Check sheet for the modelled part. Datum: model origin and axes. Units: mm. A direction names the side the tool comes from. Round coordinates to 2 decimals unless told otherwise and drop trailing zeros. Order: outer loops, then holes, each group sorted by start corner. A loop starts at its lowest first (then second) coordinate and runs counter-clockwise, first axis right, second up. Notation, with made-up numbers: (-4, 13.25) -> (46, 13.25) arc R19 ccw to (46, 17.25) -> close; hole circle Ø10 at (43, -32). An arc over 180 degrees is marked (long way). Answer in a Markdown table with one row per item. Add a question column.
1. Sectioned sample at A-A, the plane y = 40. Record the boundary of the cut face in (x, z).
2. Material ranges on L1, parallel to X at y = 39, z = 0; L2, parallel to Y at x = 2.5, z = 2.75, recorded low to high. Write a range as from..to.
3. Access from +Z, -Z, +X, -X, +Y, -Y to the whole of each face (thin tool, end or side, straight path). Record for faces 5 (the cylindrical face through (2.287, 0.256, -3.434)), 6 (the cylindrical face through (-0.867, 77.644, 3.905)), 7 (the cylindrical face through (-3.746, 78.397, -0.165)), 8 (the cylindrical face through (2.42, 3.03, 2.76)).
4. Draft check along Z on faces 1 (the cylindrical face through (-0.867, 81.264, 3.905)), 2 (the flat face through (2, 3, -2.7)), 3 (the cylindrical face through (1.99, 2.56, 2.76)), 4 (the cylindrical face through (-0.163, 4.268, 3.812)). Enter one of: +Z half, -Z half, draft (parallel to the pull), parting line (faces both ways), or undercut.
5. Depth check by flat-ended pin: P1, Ø4, axis at x = -3.5, z = 2.5, coming from the +Y side; P2, Ø0.8, axis at x = 2, y = 3, coming from the -Z side; P3, Ø5, axis at y = 37.5, z = -0.5, coming from the -X side. Enter the tip coordinate at first touch or a pass-through.
```python
from build123d import *

# Parameters (mm, degrees)
ESQUISSE3_W                  = 7.5
ESQUISSE3_H                  = 5.8
ENL_V_MAT_EXTRU_1_DEPTH      = 8
CONG_1_R                     = 0.5
ENL_V_MAT_EXTRU_2_DEPTH      = 89.206964432
ENL_V_MAT_EXTRU_2_DEPTH_BACK = 89.206964432
ESQUISSE4_R                  = 0.75
ESQUISSE5_W                  = 0.75
ESQUISSE5_H                  = 3.75
ESQUISSE5_W_2                = 2.511980861
ESQUISSE5_H_2                = 0.75
BOSS_EXTRU_1_DEPTH           = 0.2
CONG_2_R                     = 0.2
CONG_2_OF_SYM_TRIE1_R        = 0.2
ENL_V_MAT_EXTRU_3_DEPTH      = 89.410568231


with BuildPart() as part:
    # Esquisse2 → Révolution1 (revolve)
    with BuildSketch(Plane.XY):
        with BuildLine():
            Line((4.014003451, 30.213287326), (4.735996549, 20.586712674))
            ThreePointArc((4.735996549, 20.586712674), (4.746497911, 20.399868856), (4.75, 20.212762933))
            Line((4.75, 20.212762933), (4.75, 0))
            Line((4.75, 0), (1, 0))
            Line((1, 0), (1, 83.950802))
            Line((1, 83.950802), (0, 83.950802))
            Line((0, 83.950802), (0, 87.950802))
            ThreePointArc((0, 87.950802), (2.828427125, 86.779229125), (4, 83.950802))
            Line((4, 83.950802), (4, 78.650802))
            Line((4, 78.650802), (3.75, 78.650802))
            Line((3.75, 78.650802), (3.75, 78.150802))
            Line((3.75, 78.150802), (4, 78.150802))
            Line((4, 78.150802), (4, 77.150802))
            Line((4, 77.150802), (3.75, 77.150802))
            Line((3.75, 77.150802), (3.75, 76.650802))
            Line((3.75, 76.650802), (4, 76.650802))
            Line((4, 76.650802), (4, 30.587237067))
            ThreePointArc((4, 30.587237067), (4.003502089, 30.400131144), (4.014003451, 30.213287326))
        make_face()
    revolve(axis=Axis((0, 0, 0), (0, 1, 0)))

    # Esquisse3 → Enlèv. mat.-Extru.1 (cut)
    with BuildSketch(Plane.XZ):
        with Locations((1, 0)):
            Rectangle(ESQUISSE3_W, ESQUISSE3_H)
    extrude(amount=-ENL_V_MAT_EXTRU_1_DEPTH, mode=Mode.SUBTRACT)

    # Congé1
    cong_1_edges = [part.edges().sort_by_distance(p)[0] for p in [
        (-4.75, 0, 0),
    ]]
    fillet(cong_1_edges, radius=CONG_1_R)

    # Esquisse4 → Enlèv. mat.-Extru.2 (cut, two sides: drawn at the far end of the back side and taken through both)
    with BuildSketch(Plane.XY.offset(-ENL_V_MAT_EXTRU_2_DEPTH_BACK)):
        with Locations((0, 5)):
            Circle(ESQUISSE4_R)
        with BuildLine():
            Line((1.161980861, 0), (3.761980861, 0))
            Line((3.761980861, 0), (3.761980861, 2.6))
            ThreePointArc((3.761980861, 2.6), (3.000458492, 0.761522369), (1.161980861, 0))
        make_face()
        Polygon((3.761980861, 8), (4.75, 10), (4.75, 8), align=None)
    extrude(amount=ENL_V_MAT_EXTRU_2_DEPTH + ENL_V_MAT_EXTRU_2_DEPTH_BACK, mode=Mode.SUBTRACT)

    # Esquisse5 → Boss.-Extru.1 (add)
    with BuildSketch(Plane.XY.offset(-2.9)):
        with Locations((0, 1.875)):
            Rectangle(ESQUISSE5_W, ESQUISSE5_H)
        Polygon((0.618718434, 3.850951481), (1.149048519, 4.381281566), (4.027145904, 1.503184182), (3.496815818, 0.972854096), align=None)
        with Locations((2.50599043, 5)):
            Rectangle(ESQUISSE5_W_2, ESQUISSE5_H_2)
    boss_extru_1 = extrude(amount=BOSS_EXTRU_1_DEPTH)

    # Congé2
    cong_2_edges = [part.edges().sort_by_distance(p)[0] for p in [
        (2.505990431, 5.375, -2.7),
        (2.505990431, 4.625, -2.7),
        (2.588097212, 2.942232874, -2.7),
        (2.057767126, 2.411902788, -2.7),
        (-0.375, 1.875, -2.7),
        (0.375, 1.875, -2.7),
    ]]
    fillet(cong_2_edges, radius=CONG_2_R - 0.0001)  # a hair under: the kernel refuses the full size

    # Symétrie1: Boss.-Extru.1 across plane
    add(boss_extru_1.mirror(Plane.XY))

    # Congé2 of Symétrie1
    cong_2_of_sym_trie1_edges = [part.edges().sort_by_distance(p)[0] for p in [
        (2.505990431, 5.375, 2.7),
        (2.505990431, 4.625, 2.7),
        (2.588097212, 2.942232874, 2.7),
        (2.057767126, 2.411902788, 2.7),
        (-0.375, 1.875, 2.7),
        (0.375, 1.875, 2.7),
    ]]
    fillet(cong_2_of_sym_trie1_edges, radius=CONG_2_OF_SYM_TRIE1_R - 0.0001)  # a hair under: the kernel refuses the full size

    # Esquisse6 → Enlèv. mat.-Extru.3 (cut, through all)
    with BuildSketch(Plane.XY.offset(2.9)):
        with BuildLine():
            Line((4.027145904, 1.503184182), (3.658059706, 1.87227038))
            ThreePointArc((3.658059706, 1.87227038), (3.516870908, 1.49795968), (3.319930166, 1.149739748))
            Line((3.319930166, 1.149739748), (3.496815818, 0.972854096))
            Line((3.496815818, 0.972854096), (4.027145904, 1.503184182))
        make_face()
    extrude(amount=-ENL_V_MAT_EXTRU_3_DEPTH, mode=Mode.SUBTRACT)


solid = part.part
```
Answer key:
| question | item | result |
|---|---|---|
| 1 | outline | circle Ø8 at (0, 0); hole circle Ø2 at (0, 0) |
| 2 | L1 | x = -4..-1, 1..4 |
| 2 | L2 | y = 2.07..2.93, 4.69..5.31, 8..85.43 |
| 3 | face 5 | +Z, -Z, +X, -Y |
| 3 | face 6 | +Y |
| 3 | face 7 | none |
| 3 | face 8 | +X |
| 4 | face 1 | parting line |
| 4 | face 2 | undercut |
| 4 | face 3 | undercut |
| 4 | face 4 | draft |
| 5 | P1 | stops at y = 87.22 |
| 5 | P2 | stops at z = -4.47 |
| 5 | P3 | stops at x = -4 |
